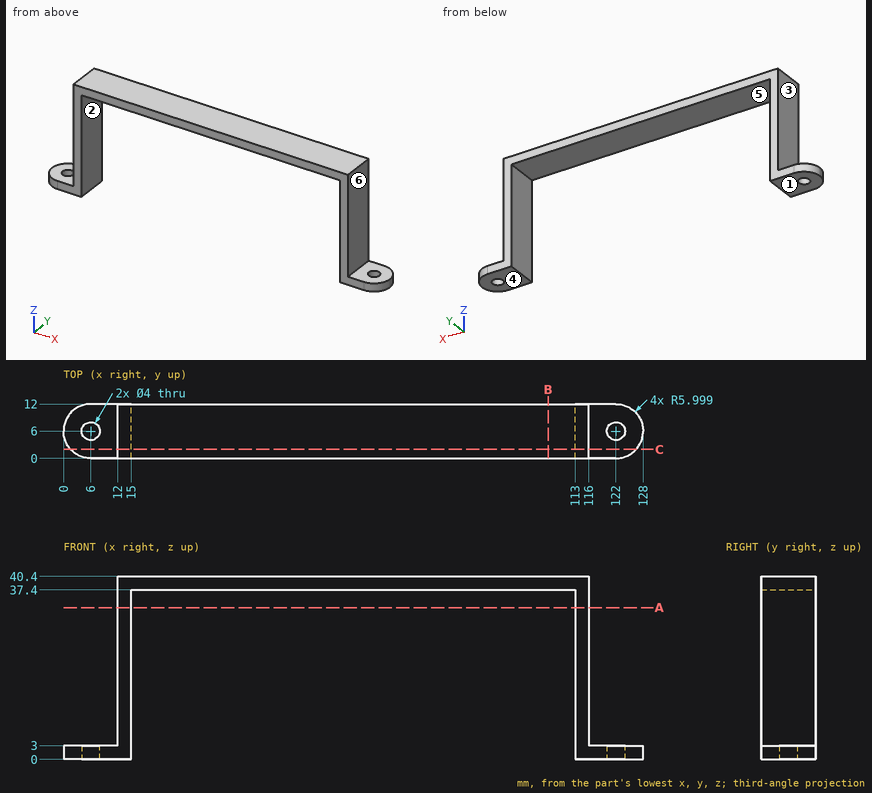
Part print with two shaded views. Sizes in mm from the minimum x, y, z corner. A direction names the side the tool comes from. Give positions to 0.01 mm unless a question says otherwise; leave off trailing zeros. Order: outer loops, then holes, each group sorted by start corner. A loop starts at its lowest first (then second) coordinate and runs counter-clockwise, first axis right, second up. Notation, with made-up numbers: M -19.5,74.5 L -10.5,74.5 A20 cw -10.5,101.5 Z; hole C -38,25.5 d11. An arc over 180 degrees is marked long. Use one line per item in the form item = value.
1) Saw through at A-A (z = 33.5). Give the cut face in (x, y), plus the area to 3 significant figures.
Calculated:
outline = M 12,0 L 15,0 L 15,12 L 12,12 Z; M 113,0 L 116,0 L 116,12 L 113,12 Z
area = 72.0 mm2
2) Tool access for the marked faces 1, 2 and 3: list every direction of +Z, -Z, +X, -X, +Y, -Y with a clear straight run to the whole face (end or side of a thin tool).
Calculated:
face_1 = -Z, +X, -X, +Y, -Y
face_2 = -Z, +Y, -Y
face_3 = +Z, -X, +Y, -Y
3) Two-plate mould, pull along X, no slides. Class the marked faces 4, 5 and 6: released by +X, released by -X, zero draft, split by the parting line, or undercut.
Calculated:
face_4 = zero draft
face_5 = undercut
face_6 = released by +X
4) Drop flat-ended pins along their axis: pin 1 (3.5 mm diameter, centred on y = 7, z = 19.5, fed in from +X); pin 2 (1.5 mm diameter, centred on x = 58, y = 5, fed in from -Z); pin 3 (6 mm diameter, centred on x = 124.5, y = 4, fed in from +Z); pin 4 (3 mm diameter, centred on x = 122, y = 6, fed in from +Z). Give the stop position or say it passes through.
Calculated:
pin_1 = 116
pin_2 = 37.4
pin_3 = 3
pin_4 = through
5) Saw through at B-B (x = 107). Give the cut face in (y, z).
Calculated:
outline = M 0,37.4 L 12,37.4 L 12,40.4 L 0,40.4 Z
6) Saw through at C-C (y = 2). Give the cut face in (x, z).
Calculated:
outline = M 1.53,0 L 15,0 L 15,37.4 L 113,37.4 L 113,0 L 126.47,0 L 126.47,3 L 116,3 L 116,40.4 L 12,40.4 L 12,3 L 1.53,3 Z
7) Probe probe 1 along X at (y, z) = (6, 2.4); probe 2 along X at (y, z) = (4.75, 26); probe 3 along Z at (x, y) = (103.5, 10.75). List the from-to ranges inside material, lowest first.
Calculated:
probe_1 = 0 to 4, 8 to 15, 113 to 120, 124 to 128
probe_2 = 12 to 15, 113 to 116
probe_3 = 37.4 to 40.4
